Part model, mm, in its own coordinate system. Coordinates: 2 decimals unless noted, no trailing zeros. Order: outer loops, then holes, each group sorted by start corner. A loop starts at its lowest first (then second) coordinate and runs counter-clockwise, first axis right, second up. Notation, with made-up numbers: (49.5, 45.5) - (65.5, 45.5) arc R7 ccw to (65.5, 49.5) - close; hole circle Ø4 at (40, 68.25). An arc over 180 degrees is marked (long way). Use a Markdown table: item, result. Add a question column.
1) Wall check: L1, parallel to X at y = -12, z = 2.7; L2, parallel to X at y = -49, z = 2.65. Give the ranges that are in metal, low to high. Write a range as [from, to].
2) Saw through at B-B on y = -13.5. List the corners of the cut face in (x, z).
3) Saw through at A-A on z = 1.25. List the corners of the cut face in (x, y), then the cut area to 3 significant figures.
4) Saw through at C-C on x = 16. List the corners of the cut face in (y, z).
5) Drop a flat-ended pin along its axis: P1, Ø1, axis at y = -17.5, z = 1.5, coming from the -X side. Give the stop position or say it passes through.
```python
from build123d import *

# Parameters (mm, degrees)
F1_DEPTH = 3


with BuildPart() as f1:
    # F0 (on Top) → F1 (new body)
    with BuildSketch(Plane.XY):
        with BuildLine():
            Line((15, 0), (0, 0))
            Line((0, 0), (-15, 0))
            Line((-15, 0), (-24.136744, -57.687131))
            ThreePointArc((-24.136744, -57.687131), (-23.682179, -59.298896), (-22.161367, -60))
            Line((-22.161367, -60), (0, -60))
            Line((0, -60), (22.161367, -60))
            ThreePointArc((22.161367, -60), (23.682179, -59.298896), (24.136744, -57.687131))
            Line((24.136744, -57.687131), (15, 0))
        make_face()
    extrude(amount=F1_DEPTH)


solid = f1.part
```
Results are:
| question | item | result |
|---|---|---|
| 1 | L1 | [-16.9, 16.9] |
| 1 | L2 | [-22.76, 22.76] |
| 2 | outline | (-17.14, 0) - (17.14, 0) - (17.14, 3) - (-17.14, 3) - close |
| 3 | outline | (-24.14, -57.69) arc R2 ccw to (-22.16, -60) - (22.16, -60) arc R2 ccw to (24.14, -57.69) - (15, 0) - (-15, 0) - close |
| 3 | area | 2,370 mm2 |
| 4 | outline | (-60, 0) - (-6.31, 0) - (-6.31, 3) - (-60, 3) - close |
| 5 | P1 | x = -17.85 |
